```python
from build123d import *

# Parameters (mm, degrees)
CHANFREIN1_SIZE         = 0.5
CHANFREIN2_SIZE         = 1
ESQUISSE2_W             = 9
ESQUISSE2_H             = 30
ENL_V_MAT_EXTRU_1_DEPTH = 30
ENL_V_MAT_EXTRU_2_REACH = 73.533
ESQUISSE3_R             = 4.1
CHANFREIN3_SIZE         = 0.5


with BuildPart() as part:
    # Esquisse1 → Révolution1 (revolve)
    with BuildSketch(Plane.XY, mode=Mode.PRIVATE) as r_volution1_sk:
        Polygon((-49, 5), (-49, 10), (0, 10), (0, 0), (-69, 0), (-69, 6), (-50, 6), (-50, 5), align=None)
    revolve(r_volution1_sk.sketch.rotate(Axis((0, 0, 0), (1, 0, 0)), 90), axis=Axis((0, 0, 0), (1, 0, 0)))

    # Chanfrein1
    chanfrein1_edges = [part.edges().sort_by_distance(p)[0] for p in [
        (-49, 0, -10),
        (0, 0, -10),
    ]]
    chamfer(chanfrein1_edges, length=CHANFREIN1_SIZE)

    # Chanfrein2
    chanfrein2_edges = [part.edges().sort_by_distance(p)[0] for p in [
        (-69, 0, -6),
    ]]
    chamfer(chanfrein2_edges, length=CHANFREIN2_SIZE)

    # Esquisse2 → Enlèv. mat.-Extru.1 (cut)
    with BuildSketch(Plane(origin=(0, 0, 0), x_dir=(0, 0, -1), z_dir=(1, 0, 0))):
        with Locations((-10.5, 0)):
            Rectangle(ESQUISSE2_W, ESQUISSE2_H)
        with Locations((10.5, 0)):
            Rectangle(ESQUISSE2_W, ESQUISSE2_H)
    extrude(amount=-ENL_V_MAT_EXTRU_1_DEPTH, mode=Mode.SUBTRACT)

    # Esquisse3 → Enlèv. mat.-Extru.2 (cut, up to next)
    with BuildSketch(Plane.XY.offset(6), mode=Mode.PRIVATE) as enl_v_mat_extru_2_sk1:
        with Locations((-11.5, 0)):
            Circle(ESQUISSE3_R)
    enl_v_mat_extru_2_tool1 = extrude(enl_v_mat_extru_2_sk1.sketch, amount=-ENL_V_MAT_EXTRU_2_REACH, mode=Mode.PRIVATE) & part.part
    add(enl_v_mat_extru_2_tool1.solids().sort_by_distance((-11.5, 0, 6))[0], mode=Mode.SUBTRACT)

    # Chanfrein3
    chanfrein3_edges = [part.edges().sort_by_distance(p)[0] for p in [
        (-15.6, 0, 6),
        (-15.6, 0, -6),
    ]]
    chamfer(chanfrein3_edges, length=CHANFREIN3_SIZE)


solid = part.part
```
Geometry check sheet. Reference: the model listing, model coordinates, mm. A direction names the side the tool comes from. Round coordinates to 2 decimals unless told otherwise and drop trailing zeros. Order: outer loops, then holes, each group sorted by start corner. A loop starts at its lowest first (then second) coordinate and runs counter-clockwise, first axis right, second up. Notation, with made-up numbers: (83, 50.25) - (133, 50.25) arc R31 cw to (133, 86.25) - close; hole circle Ø4 at (67, 26.5). An arc over 180 degrees is marked (long way). Use a Markdown table: item, result. Add a question column.
1) Mould release check, pull along Y, two halves, no side actions. Record for faces 6 (the conical face through (-0.135, 9.635, -0.092)), 7 (the flat face through (0, 0, 0)), 8 (the cylindrical face through (-49.493, -0.22, -4.995)), 9 (the cylindrical face through (-15.596, 0.18, 0.077)): released by +Y, released by -Y, zero draft, split by the parting line, or undercut.
2) Thickness scan on line 1 along Z through (x, y) = (-25, -1.5); line 2 along Y through (x, z) = (-11.5, -1.75); line 3 along X through (y, z) = (3, 7.5). Record the ranges inside material, lowest first.
3) Section check C-C (z = 0). Record the cut outline in (x, y), then the cut area to 3 significant figures.
4) Section check A-A (x = -11.5). Record the cut outline in (y, z).
5) Gauge pin test, flat ends, axial feed: P1, Ø5, axis at x = -43.5, y = -2, coming from the +Z side; P2, Ø5, axis at x = -14, y = 3, coming from the +Z side; P3, Ø1, axis at x = -33.5, y = 7, coming from the -Z side; P4, Ø1, axis at x = -57.5, y = -7.5, coming from the +Z side. Record the tip position at first contact, or that the pin passes through.
6) Section check D-D (x = -54.5). Record the cut outline in (y, z).
7) Section check B-B (y = 0). Record the cut outline in (x, z).
8) Set-up check for faces 1 (the cylindrical face through (-58.874, -1.802, 5.723)), 2 (the flat face through (-30, 0, -8)), 3 (the flat face through (-50, -4, -4)), 4 (the flat face through (-18, 0, 6)), 5 (the conical face through (-0.135, -9.635, 0.092)): record each of +Z, -Z, +X, -X, +Y, -Y from which the full face is reachable in a straight line by a thin tool's end or side.
Established:
| question | item | result |
|---|---|---|
| 1 | face 6 | released by +Y |
| 1 | face 7 | zero draft |
| 1 | face 8 | split by the parting line |
| 1 | face 9 | undercut |
| 2 | line 1 | -6 to 6 |
| 2 | line 2 | -9.85 to -4.1, 4.1 to 9.85 |
| 2 | line 3 | -49 to -30 |
| 3 | outline | (-69, -5) - (-68, -6) - (-50, -6) - (-50, -5) - (-49, -5) - (-49, -9.5) - (-48.5, -10) - (-0.5, -10) - (0, -9.5) - (0, 9.5) - (-0.5, 10) - (-48.5, 10) - (-49, 9.5) - (-49, 5) - (-50, 5) - (-50, 6) - (-68, 6) - (-69, 5) - close; hole circle Ø8.2 at (-11.5, 0) |
| 3 | area | 1,160 mm2 |
| 4 | outline | (-8, -6) - (-4.6, -6) - (-4.1, -5.5) - (-4.1, 5.5) - (-4.6, 6) - (-8, 6) arc R10 ccw to start; (4.1, -5.5) - (4.6, -6) - (8, -6) arc R10 ccw to (8, 6) - (4.6, 6) - (4.1, 5.5) - close |
| 5 | P1 | z = 10 |
| 5 | P2 | z = 6 |
| 5 | P3 | z = -7.6 |
| 5 | P4 | through |
| 6 | outline | circle Ø12 at (0, 0) |
| 7 | outline | (-69, -5) - (-68, -6) - (-50, -6) - (-50, -5) - (-49, -5) - (-49, -9.5) - (-48.5, -10) - (-30, -10) - (-30, -6) - (-16.1, -6) - (-15.6, -5.5) - (-15.6, 5.5) - (-16.1, 6) - (-30, 6) - (-30, 10) - (-48.5, 10) - (-49, 9.5) - (-49, 5) - (-50, 5) - (-50, 6) - (-68, 6) - (-69, 5) - close; (-7.4, -5.5) - (-6.9, -6) - (0, -6) - (0, 6) - (-6.9, 6) - (-7.4, 5.5) - close |
| 8 | face 1 | -X |
| 8 | face 2 | -Z, +X, +Y, -Y |
| 8 | face 3 | none |
| 8 | face 4 | +Z, +X, +Y, -Y |
| 8 | face 5 | +X, -Y |
